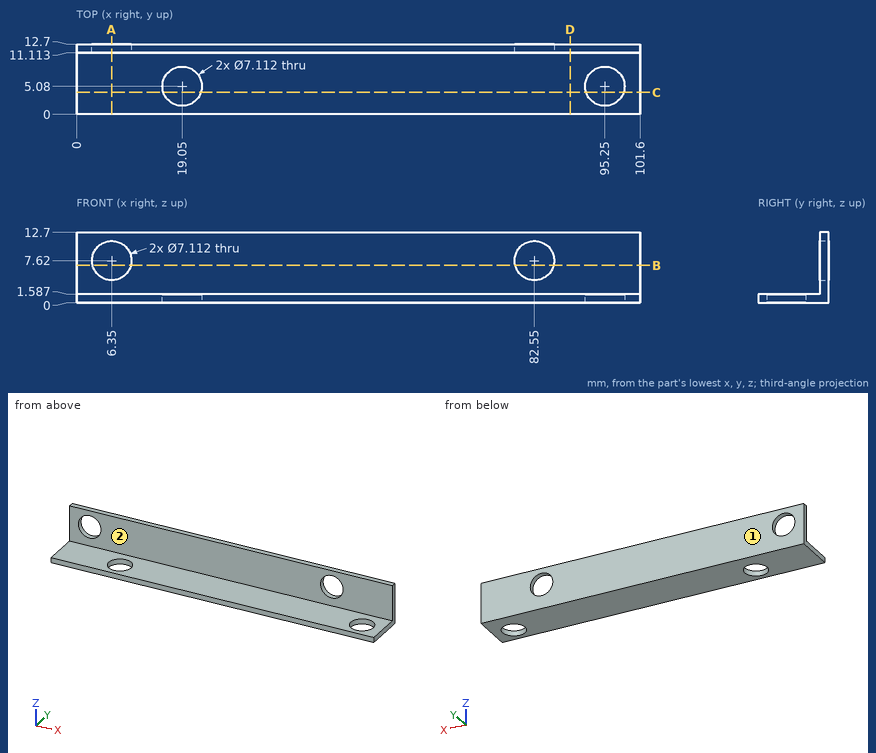
Job drawing, mm, ordinate dimensions from the low corner. One solid piece. A direction names the side the tool comes from. Give positions to 0.01 mm unless a question says otherwise; leave off trailing zeros. Loops run counter-clockwise (first coordinate to the right, second up) from the corner with the lowest first, then second, coordinate; pieces in that order, holes last. Notation, with made-up numbers: (84, 61) -> (97, 61) arc R26 ccw to (97, 82) -> close; hole circle Ø5 at (-17, 48.5). An arc over 180 degrees is marked (long way). Use a Markdown table: item, result. Add a question column.
(1) Drop flat-ended pins along their axis: pin 1 Ø1 at (x, z) = (12, 11.5) entering from -Y; pin 2 Ø4 at (y, z) = (4, 3.5) entering from +X; pin 3 Ø5.5 at (x, y) = (36, 4) entering from +Z. Give the stop position or say it passes through.
(2) Slice it at B-B on z = 6.75. List the corners of the cut face in (x, y).
(3) Slice it at C-C on y = 4. List the corners of the cut face in (x, z), and give its area (3 significant figures).
(4) Slice it at D-D on x = 89. List the corners of the cut face in (y, z).
(5) Slice it at A-A on x = 6.35. List the corners of the cut face in (y, z) (1 decimal).
(6) Tool access for the marked faces 1 and 2: list every direction of +Z, -Z, +X, -X, +Y, -Y with a clear straight run to the whole face (end or side of a thin tool).
(7) Wall check: line 1 along Y through (x, z) = (95.25, 0.5) (1 decimal); line 2 along Z through (x, y) = (6.35, 12.3) (1 decimal); line 3 along X through (y, z) = (11.5, 7). Give the ranges that are in metal, low to high.
Filled sheet:
| question | item | result |
|---|---|---|
| 1 | pin 1 | y = 11.11 |
| 1 | pin 2 | x = 101.6 |
| 1 | pin 3 | z = 1.59 |
| 2 | outline | (0, 11.11) -> (2.9, 11.11) -> (2.9, 12.7) -> (0, 12.7) -> close; (9.8, 11.11) -> (79.1, 11.11) -> (79.1, 12.7) -> (9.8, 12.7) -> close; (86, 11.11) -> (101.6, 11.11) -> (101.6, 12.7) -> (86, 12.7) -> close |
| 3 | outline | (0, 0) -> (15.66, 0) -> (15.66, 1.59) -> (0, 1.59) -> close; (22.44, 0) -> (91.86, 0) -> (91.86, 1.59) -> (22.44, 1.59) -> close; (98.64, 0) -> (101.6, 0) -> (101.6, 1.59) -> (98.64, 1.59) -> close |
| 3 | area | 140 mm2 |
| 4 | outline | (0, 0) -> (12.7, 0) -> (12.7, 12.7) -> (11.11, 12.7) -> (11.11, 1.59) -> (0, 1.59) -> close |
| 5 | outline | (0, 0) -> (12.7, 0) -> (12.7, 4.1) -> (11.1, 4.1) -> (11.1, 1.6) -> (0, 1.6) -> close; (11.1, 11.2) -> (12.7, 11.2) -> (12.7, 12.7) -> (11.1, 12.7) -> close |
| 6 | face 1 | +Z, -Z, +X, -X, +Y |
| 6 | face 2 | +Z, +X, -X, -Y |
| 7 | line 1 | 0 to 1.5, 8.6 to 12.7 |
| 7 | line 2 | 0 to 4.1, 11.2 to 12.7 |
| 7 | line 3 | 0 to 2.85, 9.85 to 79.05, 86.05 to 101.6 |
